Here's the drawing with two shaded views (mm, measured from the low corner). I have some questions. A direction names the side the tool comes from. Round coordinates to 2 decimals unless told otherwise and drop trailing zeros. Write each loop counter-clockwise with the first axis right and the second up, starting at its lowest first coordinate (ties: lowest second). Pieces come first, ordered by that corner, then holes. Notation, with made-up numbers: (75, 22) -> (106, 22) arc R29 cw to (106, 43) -> close; hole circle Ø3 at (61, -6.5). An arc over 180 degrees is marked (long way). Use CSV: the item, a comma, the result in double quotes.
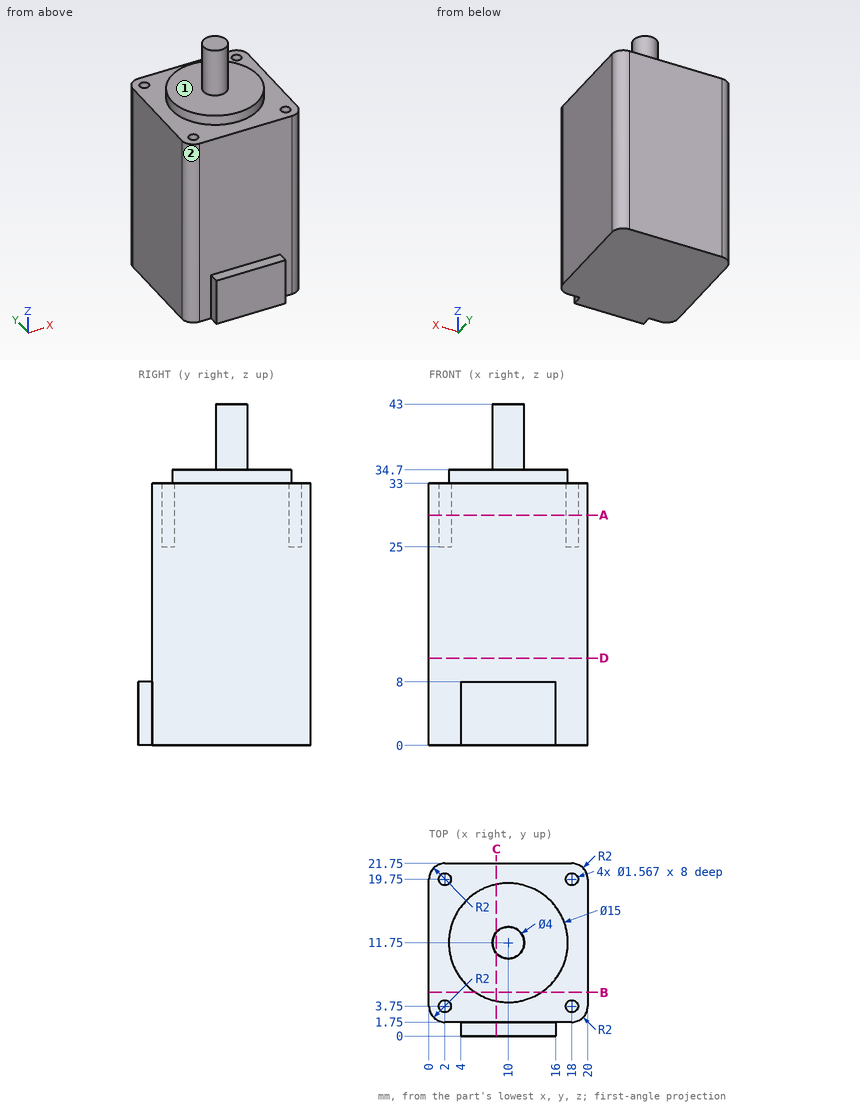
Q1. Will these pins go through, and if not, where does the flat tip stop? P1, Ø3, axis at x = 9, z = 21.5, coming from the -Y side; P2, Ø1.3, axis at x = 18, y = 4, coming from the +Z side; P3, Ø0.5, axis at y = 1, z = 3, coming from the -X side.
Resolved:
P1,"stops at y = 1.75"
P2,"stops at z = 33"
P3,"stops at x = 4"
Q2. On a 3-axis mill with a long thin cutter (end or side, diameter ignored), from which of +Z, -Z, +X, -X, +Y, -Y can I reach the whole of each face in a straight line? I mean the marked faces 1 and 2. Say none if no direction works.
Resolved:
face 1,"+Z"
face 2,"+Z, -Z, -X, -Y"
Q3. Suppose I cut it at A-A (z = 29). Write out the boundary of the cut face in (x, y).
Resolved:
outline,"(0, 3.75) arc R2 ccw to (2, 1.75) -> (18, 1.75) arc R2 ccw to (20, 3.75) -> (20, 19.75) arc R2 ccw to (18, 21.75) -> (2, 21.75) arc R2 ccw to (0, 19.75) -> close; hole circle Ø1.57 at (2, 3.75); hole circle Ø1.57 at (2, 19.75); hole circle Ø1.57 at (18, 3.75); hole circle Ø1.57 at (18, 19.75)"
Q4. Suppose I cut it at C-C (x = 8.5). Write out the boundary of the cut face in (y, z), and give its area (3 significant figures).
Resolved:
outline,"(0, 0) -> (21.75, 0) -> (21.75, 33) -> (19.1, 33) -> (19.1, 34.7) -> (13.07, 34.7) -> (13.07, 43) -> (10.43, 43) -> (10.43, 34.7) -> (4.4, 34.7) -> (4.4, 33) -> (1.75, 33) -> (1.75, 8) -> (0, 8) -> close"
area,"721 mm^2"
Q5. Suppose I cut it at B-B (y = 5.5). Write out the boundary of the cut face in (x, z).
Resolved:
outline,"(0, 0) -> (20, 0) -> (20, 33) -> (14.15, 33) -> (14.15, 34.7) -> (5.85, 34.7) -> (5.85, 33) -> (0, 33) -> close"
Q6. Suppose I cut it at D-D (z = 11). Write out the boundary of the cut face in (x, y), and give its area (3 significant figures).
Resolved:
outline,"(0, 3.75) arc R2 ccw to (2, 1.75) -> (18, 1.75) arc R2 ccw to (20, 3.75) -> (20, 19.75) arc R2 ccw to (18, 21.75) -> (2, 21.75) arc R2 ccw to (0, 19.75) -> close"
area,"397 mm^2"
Q7. Please list where these lines run through material, in increasing order: probe 1 along X at (y, z) = (3.75, 27); probe 2 along Y at (x, z) = (2, 28).
Resolved:
probe 1,"x = 0 to 1.22, 2.78 to 17.22, 18.78 to 20"
probe 2,"y = 1.75 to 2.97, 4.53 to 18.97, 20.53 to 21.75"
